For this review, take the finished solid that the model builds, in its own axes (mm). Give positions to 0.01 mm unless a question says otherwise; leave off trailing zeros. Loops run counter-clockwise (first coordinate to the right, second up) from the corner with the lowest first, then second, coordinate; pieces in that order, holes last. Notation, with made-up numbers: (6.5, 36.5) - (42.5, 36.5) arc R23 cw to (42.5, 52.5) - close; hole circle Ø9 at (-3, 28). An arc over 180 degrees is marked (long way). Answer in a Markdown table with one row per item.
```python
from build123d import *

# Parameters (mm, degrees)
SKETCH_1_R      = 5
EXTRUDE_1_DEPTH = 100
SKETCH_2_R      = 10
EXTRUDE_2_DEPTH = 2
SKETCH_3_R      = 15
SKETCH_3_R_2    = 2
EXTRUDE_3_DEPTH = 2


with BuildPart() as part:
    # 草图1 → 凸台-拉伸1 (new, symmetric)
    with BuildSketch(Plane.XY):
        Circle(SKETCH_1_R)
    extrude(amount=EXTRUDE_1_DEPTH, both=True)

    # 草图2 → 凸台-拉伸2 (add)
    with BuildSketch(Plane(origin=(0, 0, -100), x_dir=(-1, 0, 0), z_dir=(0, 0, -1))):
        Circle(SKETCH_2_R)
    extrude(amount=EXTRUDE_2_DEPTH)

    # 草图3 → 凸台-拉伸3 (add)
    with BuildSketch(Plane.XY.offset(100)):
        Circle(SKETCH_3_R)
        with Locations((-10, 0)):
            Circle(SKETCH_3_R_2, mode=Mode.SUBTRACT)
        with Locations(Location((10, 0, 0), (0, 0, 180))):
            Circle(SKETCH_3_R_2, mode=Mode.SUBTRACT)
    extrude(amount=EXTRUDE_3_DEPTH)


solid = part.part
```
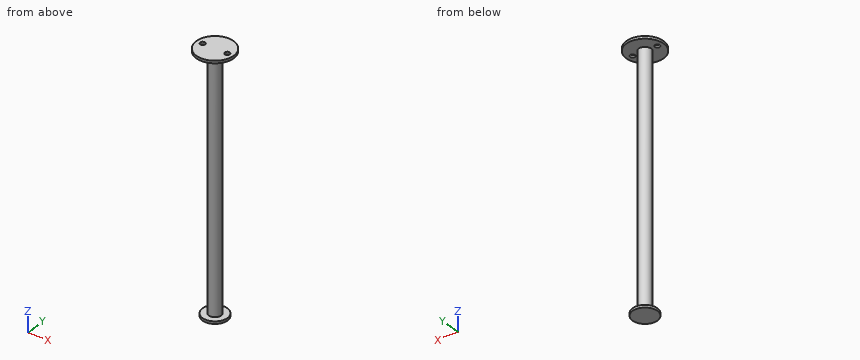
1. We need section A-A, the plane y = 0. Give the boundary of the cut face in (x, z).
Values:
| item | result |
|---|---|
| outline | (-15, 100) - (-12, 100) - (-12, 102) - (-15, 102) - close; (-10, -102) - (10, -102) - (10, -100) - (5, -100) - (5, 100) - (8, 100) - (8, 102) - (-8, 102) - (-8, 100) - (-5, 100) - (-5, -100) - (-10, -100) - close; (12, 100) - (15, 100) - (15, 102) - (12, 102) - close |
2. Wall thickness on line 1 (Z direction, x = -5.75, y = -4); line 2 (Z direction, x = -1, y = 12.5); line 3 (Y direction, x = 10, z = 100.5): over which ranges is each line inside the solid? List them lowest first. Write a range as [from, to].
Values:
| item | result |
|---|---|
| line 1 | z = [-102, -100], [100, 102] |
| line 2 | z = [100, 102] |
| line 3 | y = [-11.18, -2], [2, 11.18] |
3. Clearance check with flat-ended pins moving along their axes: pin 1 (2.5 mm diameter, centred on x = 10, y = 0, fed in from +Z); pin 2 (10 mm diameter, centred on x = 9.5, z = -6, fed in from +Y); pin 3 (3 mm diameter, centred on y = 6, z = -76.5, fed in from +X); pin 4 (4 mm diameter, centred on y = -8.5, z = 66, fed in from -X). State where each tip first meets the part, or that it passes through.
Values:
| item | result |
|---|---|
| pin 1 | stops at z = -100 |
| pin 2 | stops at y = 2.18 |
| pin 3 | stops at x = 2.18 |
| pin 4 | passes through |
4. We need section B-B, the plane x = 0. Give the boundary of the cut face in (y, z).
Values:
| item | result |
|---|---|
| outline | (-15, 100) - (-5, 100) - (-5, -100) - (-10, -100) - (-10, -102) - (10, -102) - (10, -100) - (5, -100) - (5, 100) - (15, 100) - (15, 102) - (-15, 102) - close |
5. We need section C-C, the plane z = 50.5. Give the boundary of the cut face in (x, y), and give its area (3 significant figures).
Values:
| item | result |
|---|---|
| outline | circle Ø10 at (0, 0) |
| area | 78.5 mm^2 |
